For this review, take the finished solid that the model builds, in its own axes (mm). Face numbers are marked on the shaded views. A direction names the side the tool comes from. Give positions to 0.01 mm unless a question says otherwise; leave off trailing zeros. Order: outer loops, then holes, each group sorted by start corner. A loop starts at its lowest first (then second) coordinate and runs counter-clockwise, first axis right, second up. Notation, with made-up numbers: M -19.5,-23 L 26.5,-23 A23 cw 26.5,-12 Z; hole C 88,70.25 d7. An arc over 180 degrees is marked long. Answer as CSV lines item,"result". Start each with the question number.
1. Clearance check with flat-ended pins moving along their axes: P1, Ø1.5, axis at y = 3, z = -2.5, coming from the +X side; P2, Ø2.5, axis at x = -1.5, z = 0.5, coming from the +Y side. State where each tip first meets the part, or that it passes through.
2. We need section A-A, the plane x = 0. Give the boundary of the cut face in (y, z), and give its area (3 significant figures).
3. We need section D-D, the plane y = 1.3. Give the boundary of the cut face in (x, z).
4. Machinability: for the marked faces 1 and 2, which of the approach directions +Z, -Z, +X, -X, +Y, -Y give a long, thin tool a straight path to every point of the face, cutting with its end or side? Answer none if there is none.
5. We need section B-B, the plane y = 3.05. Give the boundary of the cut face in (x, z).
6. We need section C-C, the plane z = 1.5. Give the boundary of the cut face in (x, y), and give its area (3 significant figures).
7. For line 1 along X through (y, z) = (1.9, 0); line 2 along Y through (x, z) = (-0.5, -2.75); line 3 along Z through (x, y) = (-1.25, 1.05), list the stretches that pass through material, from the lowest coordinate up.
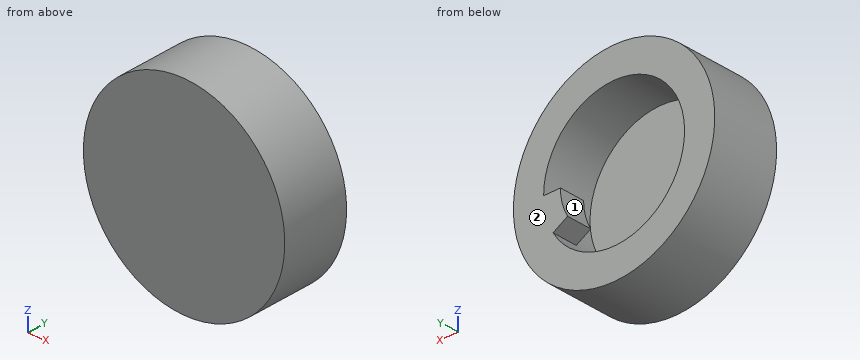
from build123d import *

# Parameters (mm, degrees)
SKETCH1_R           = 6
SKETCH1_R_2         = 4.2
BOSS_EXTRUDE1_DEPTH = 4
SKETCH1_3_R         = 6
SKETCH1_3_R_2       = 4.2
BOSS_EXTRUDE2_DEPTH = 1
BOSS_EXTRUDE3_START = 2.5
BOSS_EXTRUDE3_DEPTH = 1.5


with BuildPart() as part:
    # Sketch1 → Boss-Extrude1 (new body)
    with BuildSketch(Plane(origin=(0, 0, 0), x_dir=(1, 0, 0), z_dir=(0, 1, 0))):
        with Locations(Location((0, 0, 0), (0, 0, 270))):
            Circle(SKETCH1_R)
        with Locations(Location((0, 0, 0), (0, 0, 270))):
            Circle(SKETCH1_R_2, mode=Mode.SUBTRACT)
    extrude(amount=BOSS_EXTRUDE1_DEPTH)

    # Sketch1<3> → Boss-Extrude2 (add)
    # profile 1 of 5: a face of its own
    with BuildSketch(Plane(origin=(0, 0, 0), x_dir=(1, 0, 0), z_dir=(0, 1, 0))):
        with Locations(Location((0, 0, 0), (0, 0, 270))):
            Circle(SKETCH1_3_R)
        with Locations(Location((0, 0, 0), (0, 0, 270))):
            Circle(SKETCH1_3_R_2, mode=Mode.SUBTRACT)
    # profile 2 of 5: a face of its own
    with BuildSketch(Plane(origin=(0, 0, 0), x_dir=(1, 0, 0), z_dir=(0, 1, 0))):
        with BuildLine():
            Line((2.771281292, 1.6), (3.637306696, 2.1))
            ThreePointArc((3.637306696, 2.1), (-4.05688847, -1.087039989), (4.2, 0))
            Line((4.2, 0), (3.2, 0))
            ThreePointArc((3.2, 0), (3.090962644, 0.828220944), (2.771281292, 1.6))
        make_face()
    # profile 3 of 5: a face of its own
    with BuildSketch(Plane(origin=(0, 0, 0), x_dir=(1, 0, 0), z_dir=(0, 1, 0))):
        with BuildLine():
            ThreePointArc((4.2, 0), (4.05688847, 1.087039989), (3.637306696, 2.1))
            Line((3.637306696, 2.1), (2.771281292, 1.6))
            ThreePointArc((2.771281292, 1.6), (3.090962644, 0.828220944), (3.2, 0))
            Line((3.2, 0), (4.2, 0))
        make_face()
    # profile 4 of 5: a face of its own
    with BuildSketch(Plane(origin=(0, 0, 0), x_dir=(1, 0, 0), z_dir=(0, 1, 0))):
        with BuildLine():
            ThreePointArc((4.2, 0), (4.05688847, 1.087039989), (3.637306696, 2.1))
            Line((3.637306696, 2.1), (2.771281292, 1.6))
            ThreePointArc((2.771281292, 1.6), (3.090962644, 0.828220944), (3.2, 0))
            Line((3.2, 0), (4.2, 0))
        make_face()
    # profile 5 of 5: a face of its own
    with BuildSketch(Plane(origin=(0, 0, 0), x_dir=(1, 0, 0), z_dir=(0, 1, 0))):
        with BuildLine():
            Line((2.771281292, 1.6), (3.637306696, 2.1))
            ThreePointArc((3.637306696, 2.1), (-4.05688847, -1.087039989), (4.2, 0))
            Line((4.2, 0), (3.2, 0))
            ThreePointArc((3.2, 0), (3.090962644, 0.828220944), (2.771281292, 1.6))
        make_face()
    extrude(amount=BOSS_EXTRUDE2_DEPTH)

    # Sketch1<4> → Boss-Extrude3 (add)
    with BuildSketch(Plane(origin=(0, 0, 0), x_dir=(1, 0, 0), z_dir=(0, 1, 0)).offset(BOSS_EXTRUDE3_START)):
        with BuildLine():
            ThreePointArc((4.2, 0), (4.05688847, 1.087039989), (3.637306696, 2.1))
            Line((3.637306696, 2.1), (2.771281292, 1.6))
            ThreePointArc((2.771281292, 1.6), (3.090962644, 0.828220944), (3.2, 0))
            Line((3.2, 0), (4.2, 0))
        make_face()
    extrude(amount=BOSS_EXTRUDE3_DEPTH)


solid = part.part
Result set:
1,P1,"x = 5.74"
1,P2,"y = 1"
2,outline,"M 0,-6 L 4,-6 L 4,-4.2 L 1,-4.2 L 1,4.2 L 4,4.2 L 4,6 L 0,6 Z"
2,area,"22.8 mm2"
3,outline,"C 0,0 d12; hole C 0,0 d8.4"
4,face 1,"+Y"
4,face 2,"+Z, -Z, +X, -X, +Y"
5,outline,"C 0,0 d12; hole M 2.77,-1.6 A3.2 ccw 3.2,0 L 4.2,0 A4.2 ccw long 3.64,-2.1 Z"
6,outline,"M -5.81,0 L 5.81,0 L 5.81,4 L 3.92,4 L 3.92,1 L -3.92,1 L -3.92,4 L -5.81,4 Z"
6,area,"22.9 mm2"
7,line 1,"-6 to -4.2, 4.2 to 6"
7,line 2,"0 to 1"
7,line 3,"-5.87 to -4.01, 4.01 to 5.87"
